Geometry: final body of the model. Coordinates: model frame, mm. A direction names the side the tool comes from. Round coordinates to 2 decimals unless told otherwise and drop trailing zeros. Write each loop counter-clockwise with the first axis right and the second up, starting at its lowest first coordinate (ties: lowest second). Pieces come first, ordered by that corner, then holes. Notation, with made-up numbers: M -0.5,-30 L 21.5,-30 A11 cw 21.5,-13 Z; hole C 31.25,57 d10. An arc over 180 degrees is marked long. Use one line per item in the form item = value. Start each with the question number.
Item 1: Section query A-A (x = 46.99). Return loops of the section in (y, z) (3 decimals), and give its area (3 significant figures).
Item 2: Pull-direction query (X, two-part tool) for faces 1 (the flat face through (-27.88, -24, 2)), 2 (the flat face through (54.55, -27, 2)), 3 (the cylindrical face through (-1.1, -74.92, 1.5)); classes: pulls with the +X half, pulls with the -X half, needs draft (parallel to the pull), parting line crosses it, or undercut.
Item 3: Section query B-B (z = 2.15). State how many separate pieces and enclosed holes the cut face has, and give its area (3 significant figures).
Item 4: Ray query, probe 1 along X at (y, z) = (-45, 0.9); probe 2 along X at (y, z) = (-64, 2.9); probe 3 along X at (y, z) = (-61, 0.2). Return the intervals inside material, ascending.
Item 5: Pin query (flat end, axial travel): pin 1 Ø0.5 at (y, z) = (-26, 1.5) entering from +X; pin 2 Ø2 at (x, y) = (25.94, -45.65) entering from +Z; pin 3 Ø0.9 at (y, z) = (-29, 1) entering from -X; pin 4 Ø12 at (x, y) = (-28.5, -56.5) entering from -Z. Return the tip coordinate at first contact, or that it passes through.
Item 6: Reachability of faces 4 (the flat face through (-60, -37.338, 2)), 5 (the flat face through (60, -37.338, 2)), 6 (the cylindrical face through (1.895, -20.621, 1.545)), 7 (the flat face through (2.381, -50, 2)) from +Z, -Z, +X, -X, +Y, -Y: full face, straight path, thin tool, end or side. Return the list, or none.
from build123d import *

# Parameters (mm, degrees)
SKETCH1_R                 = 1.651
BOSS_EXTRUDE2_DEPTH       = 3.048
SKETCH2_R                 = 1.143
CUT_EXTRUDE1_DEPTH        = 4.048
SKETCH3_R                 = 12.1285
CUT_EXTRUDE2_DEPTH        = 4.048
SKETCH4_W                 = 28.562713242
SKETCH4_H                 = 11.677503754
BOSS_EXTRUDE3_DEPTH       = 3.048
SKETCH5_W                 = 216.7214489
SKETCH5_H                 = 130.569220634
CUT_EXTRUDE4_DEPTH        = 4.048
SKETCH6_W                 = 4.7625
SKETCH6_H                 = 27.432
CUT_EXTRUDE5_DEPTH        = 4.048
SKETCH10_W                = 11.43
SKETCH10_H                = 10.16
CUT_EXTRUDE9_DEPTH        = 4.048
FILLET1_R                 = 6
FILLET2_R                 = 6
SKETCH66_R                = 1.651
CUT_EXTRUDE65_DEPTH       = 97.79
SKETCH120_R               = 3.175
CUT_EXTRUDE119_DEPTH      = 103.378
CUT_EXTRUDE119_DEPTH_BACK = 48.768
CUT_EXTRUDE12_DEPTH       = 10
FILLET3_R                 = 2.54


with BuildPart() as part:
    # Sketch1 → Boss-Extrude2 (new body)
    with BuildSketch(Plane.XY):
        with BuildLine():
            Line((-64.964441474, 37.338), (-54.550441474, 37.338))
            Line((-54.550441474, 37.338), (-54.550441474, -37.338))
            Line((-54.550441474, -37.338), (-64.964441474, -37.338))
            ThreePointArc((-64.964441474, -37.338), (0, -74.93), (64.964441474, -37.338))
            Line((64.964441474, -37.338), (54.550441474, -37.338))
            Line((54.550441474, -37.338), (54.550441474, 37.338))
            Line((54.550441474, 37.338), (64.964441474, 37.338))
            ThreePointArc((64.964441474, 37.338), (0, 74.93), (-64.964441474, 37.338))
        make_face()
        with Locations((-46.482, 11.049)):
            Circle(SKETCH1_R, mode=Mode.SUBTRACT)
        with Locations((-21.083270032, 10.795)):
            Circle(SKETCH1_R, mode=Mode.SUBTRACT)
        with Locations((-21.083270032, -10.795)):
            Circle(SKETCH1_R, mode=Mode.SUBTRACT)
        with Locations((-46.482, -11.049)):
            Circle(SKETCH1_R, mode=Mode.SUBTRACT)
        with Locations((46.482, -11.049)):
            Circle(SKETCH1_R, mode=Mode.SUBTRACT)
        with Locations((21.083270032, -10.795)):
            Circle(SKETCH1_R, mode=Mode.SUBTRACT)
        with Locations((21.083270032, 10.795)):
            Circle(SKETCH1_R, mode=Mode.SUBTRACT)
        with Locations((46.482, 11.049)):
            Circle(SKETCH1_R, mode=Mode.SUBTRACT)
    extrude(amount=BOSS_EXTRUDE2_DEPTH)

    # Sketch2 → Cut-Extrude1 (cut, through all)
    with BuildSketch(Plane.XY.offset(3.048)):
        with Locations((-6.731, 62.23)):
            Circle(SKETCH2_R)
        with Locations((6.731, 62.23)):
            Circle(SKETCH2_R)
    extrude(amount=-CUT_EXTRUDE1_DEPTH, mode=Mode.SUBTRACT)

    # Sketch3 → Cut-Extrude2 (cut, through all)
    with BuildSketch(Plane(origin=(0, 0, 0), x_dir=(-1, 0, 0), z_dir=(0, 0, -1))):
        with Locations((-15.777608989, -58.882838371)):
            Circle(SKETCH3_R)
        with Locations((15.777608989, -58.882838371)):
            Circle(SKETCH3_R)
        with Locations((-43.105229381, -43.105229381)):
            Circle(SKETCH3_R)
        with Locations((19.05, 32.995567884)):
            Circle(SKETCH3_R)
        with Locations((-43.105229381, 43.105229381)):
            Circle(SKETCH3_R)
        with Locations((43.105229381, 43.105229381)):
            Circle(SKETCH3_R)
        with Locations((-19.05, 32.995567884)):
            Circle(SKETCH3_R)
        with Locations((43.105229381, -43.105229381)):
            Circle(SKETCH3_R)
    extrude(amount=-CUT_EXTRUDE2_DEPTH, mode=Mode.SUBTRACT)

    # Sketch4 → Boss-Extrude3 (add)
    with BuildSketch(Plane(origin=(0, 0, 0), x_dir=(-1, 0, 0), z_dir=(0, 0, -1))):
        with Locations((-1.488809975, 62.152540216)):
            Rectangle(SKETCH4_W, SKETCH4_H)
    extrude(amount=-BOSS_EXTRUDE3_DEPTH)

    # Sketch5 → Cut-Extrude4 (cut, through all)
    with BuildSketch(Plane(origin=(0, 0, 0), x_dir=(-1, 0, 0), z_dir=(0, 0, -1))):
        with Locations((23.316688373, 48.139610317)):
            Rectangle(SKETCH5_W, SKETCH5_H)
    extrude(amount=-CUT_EXTRUDE4_DEPTH, mode=Mode.SUBTRACT)

    # Sketch6 → Cut-Extrude5 (cut, through all)
    with BuildSketch(Plane(origin=(0, 0, 0), x_dir=(-1, 0, 0), z_dir=(0, 0, -1))):
        with Locations((0, -45.847)):
            Rectangle(SKETCH6_W, SKETCH6_H)
        Polygon((-2.38125, -34.131), (-2.38125, -32.131), (-6.38125, -32.131), (-6.38125, -17.145), (-9.38125, -17.145), (-9.38125, -34.131), align=None)
    extrude(amount=-CUT_EXTRUDE5_DEPTH, mode=Mode.SUBTRACT)

    # Sketch10 → Cut-Extrude9 (cut, through all)
    with BuildSketch(Plane(origin=(0, 0, 0), x_dir=(-1, 0, 0), z_dir=(0, 0, -1))):
        with Locations((-33.595441474, -22.225)):
            Rectangle(SKETCH10_W, SKETCH10_H)
        with Locations((33.595441474, -22.225)):
            Rectangle(SKETCH10_W, SKETCH10_H)
    extrude(amount=-CUT_EXTRUDE9_DEPTH, mode=Mode.SUBTRACT)

    # Fillet1
    fillet1_edges = [part.edges().sort_by_distance(p)[0] for p in [
        (6.38125, -32.131, 1.524),
    ]]
    fillet(fillet1_edges, radius=FILLET1_R)

    # Fillet2
    fillet2_edges = [part.edges().sort_by_distance(p)[0] for p in [
        (2.38125, -34.131, 1.524),
    ]]
    fillet(fillet2_edges, radius=FILLET2_R)

    # Sketch66 → Cut-Extrude65 (cut)
    with BuildSketch(Plane(origin=(30.092005081, 4.08352975, -16.1925), x_dir=(-1, 0, 0), z_dir=(0, 0, -1))):
        with Locations((4.154396091, -49.728759131)):
            Circle(SKETCH66_R)
        with Locations((56.02961407, -49.728759131)):
            Circle(SKETCH66_R)
    extrude(amount=-CUT_EXTRUDE65_DEPTH, mode=Mode.SUBTRACT)

    # Sketch120 → Cut-Extrude119 (cut, two sides)
    with BuildSketch(Plane(origin=(30.092005081, 4.08352975, 19.939), x_dir=(-1, 0, 0), z_dir=(0, 0, -1))) as cut_extrude119_sk:
        with Locations((77.082005081, -29.48352975)):
            Circle(SKETCH120_R)
        with Locations((30.092005081, -29.48352975)):
            Circle(SKETCH120_R)
        with Locations((-16.897994919, -29.48352975)):
            Circle(SKETCH120_R)
    extrude(amount=CUT_EXTRUDE119_DEPTH, mode=Mode.SUBTRACT)
    extrude(cut_extrude119_sk.sketch, amount=-CUT_EXTRUDE119_DEPTH_BACK, mode=Mode.SUBTRACT)

    # Sketch13 → Cut-Extrude12 (cut)
    with BuildSketch(Plane(origin=(0, 0, 0), x_dir=(-1, 0, 0), z_dir=(0, 0, -1))):
        with BuildLine():
            Line((-12.7, -20.24), (-8.888991966, -20.24))
            ThreePointArc((-8.888991966, -20.24), (-5.715, -23.495), (-2.541008034, -20.24))
            Line((-2.541008034, -20.24), (2.541008034, -20.24))
            ThreePointArc((2.541008034, -20.24), (5.715, -23.495), (8.888991966, -20.24))
            Line((8.888991966, -20.24), (12.7, -20.24))
            ThreePointArc((12.7, -20.24), (16.235533906, -11.704466094), (7.7, -15.24))
            Line((7.7, -15.24), (-1.0625, -15.24))
            ThreePointArc((-1.0625, -15.24), (-4.012347567, -10.679640913), (-9.38125, -11.500227489))
            ThreePointArc((-9.38125, -11.500227489), (-17.374337523, -13.465015853), (-12.7, -20.24))
        make_face()
    extrude(amount=-CUT_EXTRUDE12_DEPTH, mode=Mode.SUBTRACT)

    # Fillet3
    fillet3_edges = [part.edges().sort_by_distance(p)[0] for p in [
        (39.310441474, -17.145, 1.524),
        (27.880441474, -17.145, 1.524),
        (-27.880441474, -17.145, 1.524),
        (-39.310441474, -17.145, 1.524),
        (6.38125, -23.424309253, 1.524),
        (9.38125, -20.24, 1.524),
        (17.322875188, -17.145, 1.524),
        (-17.322875188, -17.145, 1.524),
        (-8.888991966, -20.24, 1.524),
        (-2.541008034, -20.24, 1.524),
        (2.541008034, -20.24, 1.524),
    ]]
    fillet(fillet3_edges, radius=FILLET3_R)


solid = part.part
Working result:
q1.outline = M -58.365,0 L -54.595,0 L -54.595,3.048 L -58.365,3.048 Z; M -31.616,0 L -28.575,0 L -28.575,3.048 L -31.616,3.048 Z; M -22.225,0 L -17.145,0 L -17.145,3.048 L -22.225,3.048 Z
q1.area = 36.2 mm²
q2.face_1 = undercut
q2.face_2 = pulls with the +X half
q2.face_3 = parting line crosses it
q3.separate_pieces = 1
q3.enclosed_holes = 9
q3.area = 3,140 mm²
q4.probe_1 = -59.91 to -55.08, -31.13 to -27.46, -24.42 to -2.38, 2.38 to 24.42, 27.46 to 31.13, 55.08 to 59.91
q4.probe_2 = -38.97 to -26.77, -4.78 to 4.78, 26.77 to 38.97
q4.probe_3 = -43.51 to -27.72, -3.84 to 3.84, 27.72 to 43.51
q5.pin_1 = 54.55
q5.pin_2 = through
q5.pin_3 = -54.55
q5.pin_4 = 0
q6.face_4 = +Z, -Z, -X, +Y
q6.face_5 = +Z, -Z, +X, +Y
q6.face_6 = +Z, -Z, +Y
q6.face_7 = +Z, -Z
